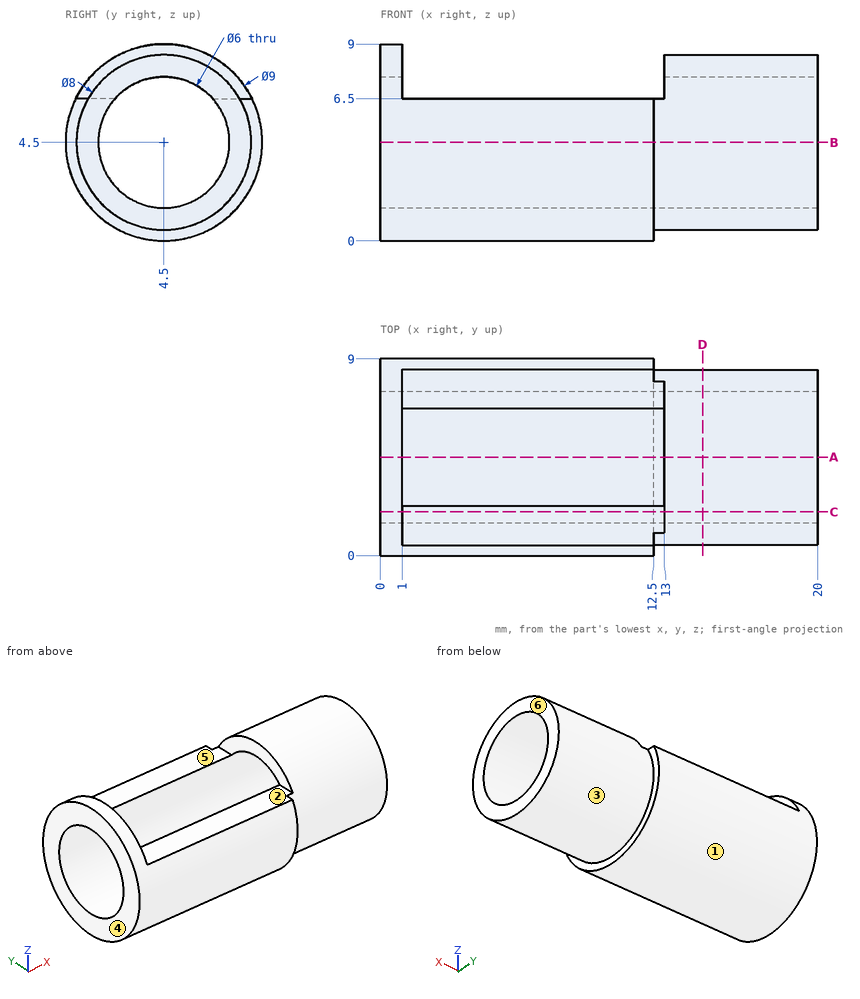
Verification items for this drawing (mm, ordinates from the low corner). A direction names the side the tool comes from. Give positions to 0.01 mm unless a question says otherwise; leave off trailing zeros. Write each loop counter-clockwise with the first axis right and the second up, starting at its lowest first coordinate (ties: lowest second). Pieces come first, ordered by that corner, then holes. Notation, with made-up numbers: (-26, 85) -> (11, 85) arc R8 cw to (11, 89) -> close; hole circle Ø6 at (-23.5, 46). An arc over 180 degrees is marked (long way). Use one line per item in the form item = value.
Item 1: Sectioned sample at A-A on y = 4.5. Enter the section's corners in (x, z).
Results list:
outline = (0, 0) -> (12.5, 0) -> (12.5, 0.5) -> (20, 0.5) -> (20, 1.5) -> (0, 1.5) -> close; (0, 7.5) -> (1, 7.5) -> (1, 9) -> (0, 9) -> close; (13, 7.5) -> (20, 7.5) -> (20, 8.5) -> (13, 8.5) -> close
Item 2: Depth check by flat-ended pin: pin 1 Ø4 at (y, z) = (5, 3.5) entering from +X; pin 2 Ø2 at (x, y) = (9, 7.5) entering from +Z; pin 3 Ø2 at (x, y) = (14, 4) entering from -Z; pin 4 Ø4 at (x, y) = (8.5, 7) entering from -Z. Enter the tip coordinate at first touch or a pass-through.
Results list:
pin_1 = 20
pin_2 = 6.5
pin_3 = 0.5
pin_4 = 0.03
Item 3: Sectioned sample at C-C on y = 2. Enter the section's corners in (x, z), plus the area to 3 significant figures.
Results list:
outline = (0, 0.76) -> (12.5, 0.76) -> (12.5, 1.38) -> (20, 1.38) -> (20, 2.84) -> (0, 2.84) -> close; (0, 6.16) -> (20, 6.16) -> (20, 7.62) -> (13, 7.62) -> (13, 6.5) -> (1, 6.5) -> (1, 8.24) -> (0, 8.24) -> close
area = 53.5 mm2
Item 4: Scan lines: line 1 (X direction, y = 4.75, z = 8); line 2 (Z direction, x = 13.25, y = 4.5); line 3 (Y direction, x = 6, z = 5.75). Record each from-to range of solid material in increasing order.
Results list:
line_1 = 0 to 1, 13 to 20
line_2 = 0.5 to 1.5, 7.5 to 8.5
line_3 = 0.18 to 1.77, 7.23 to 8.82
Item 5: Sectioned sample at B-B on z = 4.5. Enter the section's corners in (x, y), plus the area to 3 significant figures.
Results list:
outline = (0, 0) -> (12.5, 0) -> (12.5, 0.5) -> (20, 0.5) -> (20, 1.5) -> (0, 1.5) -> close; (0, 7.5) -> (20, 7.5) -> (20, 8.5) -> (12.5, 8.5) -> (12.5, 9) -> (0, 9) -> close
area = 52.5 mm2
Item 6: Access from +Z, -Z, +X, -X, +Y, -Y to the whole of each face (thin tool, end or side, straight path). Record for the marked faces 1 and 2.
Results list:
face_1 = +X, -X
face_2 = +Z, +Y, -Y
Item 7: Sectioned sample at D-D on x = 14.75. Enter the section's corners in (y, z).
Results list:
outline = circle Ø8 at (4.5, 4.5); hole circle Ø6 at (4.5, 4.5)
Item 8: Mould release check, pull along X, two halves, no side actions. Record for the marked faces 3, 4, 5 and 6: released by +X, released by -X, zero draft, split by the parting line, or undercut.
Results list:
face_3 = zero draft
face_4 = released by -X
face_5 = undercut
face_6 = released by +X
